For this review, take the finished solid that the model builds, in its own axes (mm). Face numbers are marked on the shaded views. A direction names the side the tool comes from. Coordinates: 2 decimals unless noted, no trailing zeros. Loops run counter-clockwise (first coordinate to the right, second up) from the corner with the lowest first, then second, coordinate; pieces in that order, holes last.
1. Machinability: for the marked faces 1 and 2, which of the approach directions +Z, -Z, +X, -X, +Y, -Y give a long, thin tool a straight path to every point of the face, cutting with its end or side? Answer none if there is none.
2. Clearance check with flat-ended pins moving along their axes: P1, Ø2, axis at y = 15.5, z = 1.5, coming from the -X side; P2, Ø1.5, axis at y = 6, z = 6, coming from the -X side; P3, Ø5, axis at x = 17, y = 0, coming from the +Z side; P4, Ø3.5, axis at x = 0, y = -17, coming from the -Z side. State where each tip first meets the part, or that it passes through.
3. Take a section at A-A, the plane x = -17. State the section outline as (y, z) points, then the cut area to 3 significant figures.
4. To check wall thickness, follow probe 1 along Y at (x, z) = (-0.5, 0.5); probe 2 along X at (y, z) = (-4.5, 8.5); probe 3 along Y at (x, z) = (0.5, 8.5). State the ranges of each line that lie inside material, in increasing order.
5. Take a section at D-D, the plane x = -9. State the section outline as (y, z) points.
6. Take a section at C-C, the plane z = 3.5. Count the separate pieces of the cut face and the enclosed holes in it, then the cut area to 3 significant figures.
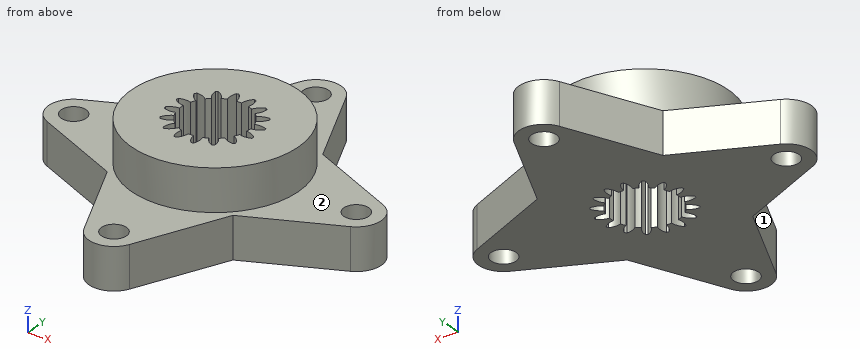
```python
from build123d import *

# Parameters (mm, degrees)
CROQUIS1_R                 = 10
CROQUIS1_R_2               = 2
SALIENTE_EXTRUIR1_DEPTH    = 10
CORTAR_EXTRUIR1_DEPTH      = 10
CORTAR_EXTRUIR1_DEPTH_BACK = 20
CROQUIS3_R                 = 1.5
CROQUIS3_R_2               = 10
SALIENTE_EXTRUIR2_DEPTH    = 5


with BuildPart() as part:
    # Croquis1 → Saliente-Extruir1 (new body)
    with BuildSketch(Plane.XY):
        Circle(CROQUIS1_R)
        Circle(CROQUIS1_R_2, mode=Mode.SUBTRACT)
    extrude(amount=SALIENTE_EXTRUIR1_DEPTH)

    # Croquis2 → Cortar-Extruir1 (cut, two sides: drawn at the far end of the back side and taken through both)
    with BuildSketch(Plane.XY.offset(10).offset(-CORTAR_EXTRUIR1_DEPTH_BACK)):
        with BuildLine():
            Line((0.91835658, 5.32133641), (1.187936434, 5.267713643))
            ThreePointArc((1.187936434, 5.267713643), (1.356901071, 4.56513254), (1.254199065, 3.849855284))
            ThreePointArc((1.254199065, 3.849855284), (1.549485218, 3.740788227), (1.835406113, 3.609111442))
            ThreePointArc((1.835406113, 3.609111442), (2.268562227, 4.187510125), (2.88483813, 4.564833947))
            Line((2.88483813, 4.564833947), (3.113376895, 4.412129226))
            ThreePointArc((3.113376895, 4.412129226), (3.000613717, 3.698368958), (2.63200468, 3.076841296))
            ThreePointArc((2.63200468, 3.076841296), (2.863075357, 2.863075357), (3.076841296, 2.63200468))
            ThreePointArc((3.076841296, 2.63200468), (3.698368958, 3.000613717), (4.412129226, 3.113376895))
            Line((4.412129226, 3.113376895), (4.564833947, 2.88483813))
            ThreePointArc((4.564833947, 2.88483813), (4.187510125, 2.268562227), (3.609111442, 1.835406113))
            ThreePointArc((3.609111442, 1.835406113), (3.740788227, 1.549485218), (3.849855284, 1.254199065))
            ThreePointArc((3.849855284, 1.254199065), (4.56513254, 1.356901071), (5.267713643, 1.187936434))
            Line((5.267713643, 1.187936434), (5.32133641, 0.91835658))
            ThreePointArc((5.32133641, 0.91835658), (4.736896076, 0.493387462), (4.036763703, 0.314546988))
            ThreePointArc((4.036763703, 0.314546988), (4.049, 0), (4.036763703, -0.314546988))
            ThreePointArc((4.036763703, -0.314546988), (4.736896076, -0.493387462), (5.32133641, -0.91835658))
            Line((5.32133641, -0.91835658), (5.267713643, -1.187936434))
            ThreePointArc((5.267713643, -1.187936434), (4.56513254, -1.356901071), (3.849855284, -1.254199065))
            ThreePointArc((3.849855284, -1.254199065), (3.740788227, -1.549485218), (3.609111442, -1.835406113))
            ThreePointArc((3.609111442, -1.835406113), (4.187510125, -2.268562227), (4.564833947, -2.88483813))
            Line((4.564833947, -2.88483813), (4.412129226, -3.113376895))
            ThreePointArc((4.412129226, -3.113376895), (3.698368958, -3.000613717), (3.076841296, -2.63200468))
            ThreePointArc((3.076841296, -2.63200468), (2.863075357, -2.863075357), (2.63200468, -3.076841296))
            ThreePointArc((2.63200468, -3.076841296), (3.000613717, -3.698368958), (3.113376895, -4.412129226))
            Line((3.113376895, -4.412129226), (2.88483813, -4.564833947))
            ThreePointArc((2.88483813, -4.564833947), (2.268562227, -4.187510125), (1.835406113, -3.609111442))
            ThreePointArc((1.835406113, -3.609111442), (1.549485218, -3.740788227), (1.254199065, -3.849855284))
            ThreePointArc((1.254199065, -3.849855284), (1.356901071, -4.56513254), (1.187936434, -5.267713643))
            Line((1.187936434, -5.267713643), (0.91835658, -5.32133641))
            ThreePointArc((0.91835658, -5.32133641), (0.493387462, -4.736896076), (0.314546988, -4.036763703))
            ThreePointArc((0.314546988, -4.036763703), (0, -4.049), (-0.314546988, -4.036763703))
            ThreePointArc((-0.314546988, -4.036763703), (-0.493387462, -4.736896076), (-0.91835658, -5.32133641))
            Line((-0.91835658, -5.32133641), (-1.187936434, -5.267713643))
            ThreePointArc((-1.187936434, -5.267713643), (-1.356901071, -4.56513254), (-1.254199065, -3.849855284))
            ThreePointArc((-1.254199065, -3.849855284), (-1.549485218, -3.740788227), (-1.835406113, -3.609111442))
            ThreePointArc((-1.835406113, -3.609111442), (-2.268562227, -4.187510125), (-2.88483813, -4.564833947))
            Line((-2.88483813, -4.564833947), (-3.113376895, -4.412129226))
            ThreePointArc((-3.113376895, -4.412129226), (-3.000613717, -3.698368958), (-2.63200468, -3.076841296))
            ThreePointArc((-2.63200468, -3.076841296), (-2.863075357, -2.863075357), (-3.076841296, -2.63200468))
            ThreePointArc((-3.076841296, -2.63200468), (-3.698368958, -3.000613717), (-4.412129226, -3.113376895))
            Line((-4.412129226, -3.113376895), (-4.564833947, -2.88483813))
            ThreePointArc((-4.564833947, -2.88483813), (-4.187510125, -2.268562227), (-3.609111442, -1.835406113))
            ThreePointArc((-3.609111442, -1.835406113), (-3.740788227, -1.549485218), (-3.849855284, -1.254199065))
            ThreePointArc((-3.849855284, -1.254199065), (-4.56513254, -1.356901071), (-5.267713643, -1.187936434))
            Line((-5.267713643, -1.187936434), (-5.32133641, -0.91835658))
            ThreePointArc((-5.32133641, -0.91835658), (-4.736896076, -0.493387462), (-4.036763703, -0.314546988))
            ThreePointArc((-4.036763703, -0.314546988), (-4.049, 0), (-4.036763703, 0.314546988))
            ThreePointArc((-4.036763703, 0.314546988), (-4.736896076, 0.493387462), (-5.32133641, 0.91835658))
            Line((-5.32133641, 0.91835658), (-5.267713643, 1.187936434))
            ThreePointArc((-5.267713643, 1.187936434), (-4.56513254, 1.356901071), (-3.849855284, 1.254199065))
            ThreePointArc((-3.849855284, 1.254199065), (-3.740788227, 1.549485218), (-3.609111442, 1.835406113))
            ThreePointArc((-3.609111442, 1.835406113), (-4.187510125, 2.268562227), (-4.564833947, 2.88483813))
            Line((-4.564833947, 2.88483813), (-4.412129226, 3.113376895))
            ThreePointArc((-4.412129226, 3.113376895), (-3.698368958, 3.000613717), (-3.076841296, 2.63200468))
            ThreePointArc((-3.076841296, 2.63200468), (-2.863075357, 2.863075357), (-2.63200468, 3.076841296))
            ThreePointArc((-2.63200468, 3.076841296), (-3.000613717, 3.698368958), (-3.113376895, 4.412129226))
            Line((-3.113376895, 4.412129226), (-2.88483813, 4.564833947))
            ThreePointArc((-2.88483813, 4.564833947), (-2.268562227, 4.187510125), (-1.835406113, 3.609111442))
            ThreePointArc((-1.835406113, 3.609111442), (-1.549485218, 3.740788227), (-1.254199065, 3.849855284))
            ThreePointArc((-1.254199065, 3.849855284), (-1.356901071, 4.56513254), (-1.187936434, 5.267713643))
            Line((-1.187936434, 5.267713643), (-0.91835658, 5.32133641))
            ThreePointArc((-0.91835658, 5.32133641), (-0.493387462, 4.736896076), (-0.314546988, 4.036763703))
            ThreePointArc((-0.314546988, 4.036763703), (0, 4.049), (0.314546988, 4.036763703))
            ThreePointArc((0.314546988, 4.036763703), (0.493387462, 4.736896076), (0.91835658, 5.32133641))
        make_face()
    extrude(amount=CORTAR_EXTRUIR1_DEPTH + CORTAR_EXTRUIR1_DEPTH_BACK, mode=Mode.SUBTRACT)

    # Croquis3 → Saliente-Extruir2 (add)
    with BuildSketch(Plane(origin=(0, 0, 0), x_dir=(-1, 0, 0), z_dir=(0, 0, -1))):
        with BuildLine():
            Line((-2.733870597, 18.235294118), (-7.558265316, 7.558265316))
            Line((-7.558265316, 7.558265316), (-18.235294118, 2.733870597))
            ThreePointArc((-18.235294118, 2.733870597), (-20, 0), (-18.235294118, -2.733870597))
            Line((-18.235294118, -2.733870597), (-7.558265316, -7.558265316))
            Line((-7.558265316, -7.558265316), (-2.733870597, -18.235294118))
            ThreePointArc((-2.733870597, -18.235294118), (0, -20), (2.733870597, -18.235294118))
            Line((2.733870597, -18.235294118), (7.558265316, -7.558265316))
            Line((7.558265316, -7.558265316), (18.235294118, -2.733870597))
            ThreePointArc((18.235294118, -2.733870597), (20, 0), (18.235294118, 2.733870597))
            Line((18.235294118, 2.733870597), (7.558265316, 7.558265316))
            Line((7.558265316, 7.558265316), (2.733870597, 18.235294118))
            ThreePointArc((2.733870597, 18.235294118), (0, 20), (-2.733870597, 18.235294118))
        make_face()
        with Locations((0, 17)):
            Circle(CROQUIS3_R, mode=Mode.SUBTRACT)
        with Locations((17, 0)):
            Circle(CROQUIS3_R, mode=Mode.SUBTRACT)
        Circle(CROQUIS3_R_2, mode=Mode.SUBTRACT)
        with Locations((0, -17)):
            Circle(CROQUIS3_R, mode=Mode.SUBTRACT)
        with Locations((-17, 0)):
            Circle(CROQUIS3_R, mode=Mode.SUBTRACT)
    extrude(amount=-SALIENTE_EXTRUIR2_DEPTH)


solid = part.part
```
Results list:
1. face 1: +Z, -Z, -X, -Y
1. face 2: +Z
2. P1: stops at x = -4.42
2. P2: stops at x = -8.51
2. P3: stops at z = 5
2. P4: stops at z = 0
3. outline: (-3.29, 0) - (-1.5, 0) - (-1.5, 5) - (-3.29, 5) - close; (1.5, 0) - (3.29, 0) - (3.29, 5) - (1.5, 5) - close
3. area: 17.9 mm2
4. probe 1: y = -19.96 to -18.41, -15.59 to -4.75, 4.75 to 15.59, 18.41 to 19.96
4. probe 2: x = -8.93 to -2.98, -2.73 to -1.36, -0.4 to 0.4, 1.36 to 2.73, 2.98 to 8.93
4. probe 3: y = -9.99 to -4.75, 4.75 to 9.99
5. outline: (-6.91, 0) - (6.91, 0) - (6.91, 5) - (4.36, 5) - (4.36, 10) - (-4.36, 10) - (-4.36, 5) - (-6.91, 5) - close
6. separate pieces: 1
6. enclosed holes: 5
6. area: 599 mm2
